from build123d import *

# Parameters (mm, degrees)
SKETCH1_R                        = 127
SKETCH1_R_2                      = 25.4
BOSS_EXTRUDE2_DEPTH              = 19.05
F_1_4_20_TAPPED_HOLE1_AT_2_COUNT = 2
F_1_4_20_TAPPED_HOLE1_AT_2_PITCH = 127
F_1_4_20_TAPPED_HOLE1_AT_3_COUNT = 2
F_1_4_20_TAPPED_HOLE1_AT_3_PITCH = 107.763073453
F_1_4_20_TAPPED_HOLE1_AT_4_COUNT = 2
F_1_4_20_TAPPED_HOLE1_AT_4_PITCH = 177.8
F_1_4_20_TAPPED_HOLE1_AT_5_COUNT = 2
F_1_4_20_TAPPED_HOLE1_AT_5_PITCH = 152.4
F_1_4_20_TAPPED_HOLE1_AT_6_COUNT = 2
F_1_4_20_TAPPED_HOLE1_AT_6_PITCH = 127
F_1_4_20_TAPPED_HOLE1_AT_7_COUNT = 2
F_1_4_20_TAPPED_HOLE1_AT_7_PITCH = 107.763073453
F_1_4_20_TAPPED_HOLE1_AT_8_COUNT = 2
F_1_4_20_TAPPED_HOLE1_AT_8_PITCH = 25.4


with BuildPart() as part:
    # Sketch1 → Boss-Extrude2 (new body)
    with BuildSketch(Plane.XY):
        Circle(SKETCH1_R)
        Circle(SKETCH1_R_2, mode=Mode.SUBTRACT)
    extrude(amount=BOSS_EXTRUDE2_DEPTH)

    # Sketch5 → 1/4-20 Tapped Hole1 (revolve, cut)
    with BuildSketch(Plane(origin=(-76.2, 0, 19.05), x_dir=(0, -1, 0), z_dir=(1, 0, 0))):
        Polygon((0, 0), (0, 19.05), (3.81, 19.05), (2.5527, 17.7927), (2.5527, 1.2573), (3.81, 0), align=None)
    f_1_4_20_tapped_hole1 = revolve(axis=Axis((-76.2, 0, 25.4), (0, 0, -1)), mode=Mode.SUBTRACT)

    # 1/4-20 Tapped Hole1 at 2: 1/4-20 Tapped Hole1 ×2
    with Locations(*[Vector(0.6, 0.8, 0) * (i * F_1_4_20_TAPPED_HOLE1_AT_2_PITCH) for i in range(1, F_1_4_20_TAPPED_HOLE1_AT_2_COUNT)]):
        add(f_1_4_20_tapped_hole1, mode=Mode.SUBTRACT)

    # 1/4-20 Tapped Hole1 at 3: 1/4-20 Tapped Hole1 ×2
    with Locations(*[Vector(0.707106781, 0.707106781, 0) * (i * F_1_4_20_TAPPED_HOLE1_AT_3_PITCH) for i in range(1, F_1_4_20_TAPPED_HOLE1_AT_3_COUNT)]):
        add(f_1_4_20_tapped_hole1, mode=Mode.SUBTRACT)

    # 1/4-20 Tapped Hole1 at 4: 1/4-20 Tapped Hole1 ×2
    with Locations(*[(i * F_1_4_20_TAPPED_HOLE1_AT_4_PITCH, 0, 0) for i in range(1, F_1_4_20_TAPPED_HOLE1_AT_4_COUNT)]):
        add(f_1_4_20_tapped_hole1, mode=Mode.SUBTRACT)

    # 1/4-20 Tapped Hole1 at 5: 1/4-20 Tapped Hole1 ×2
    with Locations(*[(i * F_1_4_20_TAPPED_HOLE1_AT_5_PITCH, 0, 0) for i in range(1, F_1_4_20_TAPPED_HOLE1_AT_5_COUNT)]):
        add(f_1_4_20_tapped_hole1, mode=Mode.SUBTRACT)

    # 1/4-20 Tapped Hole1 at 6: 1/4-20 Tapped Hole1 ×2
    with Locations(*[Vector(0.6, -0.8, 0) * (i * F_1_4_20_TAPPED_HOLE1_AT_6_PITCH) for i in range(1, F_1_4_20_TAPPED_HOLE1_AT_6_COUNT)]):
        add(f_1_4_20_tapped_hole1, mode=Mode.SUBTRACT)

    # 1/4-20 Tapped Hole1 at 7: 1/4-20 Tapped Hole1 ×2
    with Locations(*[Vector(0.707106781, -0.707106781, 0) * (i * F_1_4_20_TAPPED_HOLE1_AT_7_PITCH) for i in range(1, F_1_4_20_TAPPED_HOLE1_AT_7_COUNT)]):
        add(f_1_4_20_tapped_hole1, mode=Mode.SUBTRACT)

    # 1/4-20 Tapped Hole1 at 8: 1/4-20 Tapped Hole1 ×2
    with Locations(*[(-i * F_1_4_20_TAPPED_HOLE1_AT_8_PITCH, 0, 0) for i in range(1, F_1_4_20_TAPPED_HOLE1_AT_8_COUNT)]):
        add(f_1_4_20_tapped_hole1, mode=Mode.SUBTRACT)


solid = part.part
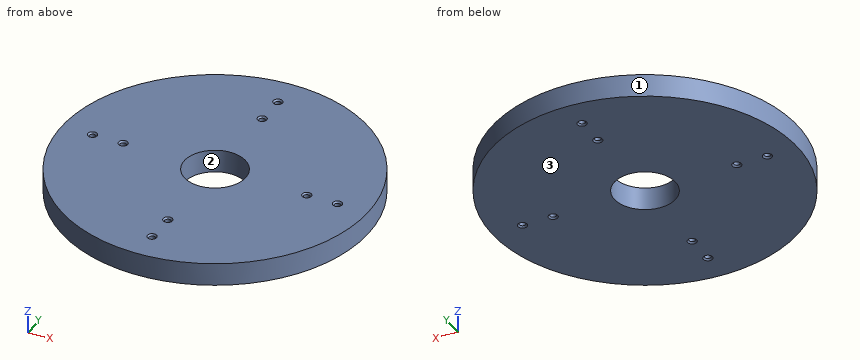
Check sheet for the modelled part. Datum: model origin and axes. Units: mm. Face numbers are marked on the shaded views. Round coordinates to 2 decimals unless told otherwise and drop trailing zeros. Loops run counter-clockwise (first coordinate to the right, second up) from the corner with the lowest first, then second, coordinate; pieces in that order, holes last. Notation, with made-up numbers: (35.5, 11) - (56.5, 11) arc R14 cw to (56.5, 26) - close; hole circle Ø6 at (-29, 26). An arc over 180 degrees is marked (long way). Answer as CSV lines item,"result". Start each with the question number.
Item 1: Release check for a two-part mould opening along Y. For the marked faces 1, 2 and 3 record: +Y half, -Y half, draft (parallel to the pull), parting line (faces both ways), or undercut.
Item 2: Scan lines: line 1 (Y direction, x = 0, z = 6.75); line 2 (X direction, y = 101.6, z = 6.25); line 3 (Y direction, x = 75, z = 13). Record each from-to range of solid material in increasing order. Write a range as [from, to].
Item 3: Section check C-C (y = 35). Record the boundary of the cut face in (x, z), and give its area (3 significant figures).
Item 4: Section check B-B (x = -22.5). Record the boundary of the cut face in (y, z).
Item 5: Section check A-A (z = 7.75). Count the separate pieces of the cut face and the enclosed holes in it, and give its area (3 significant figures).
Item 6: Depth check by flat-ended pin: P1, Ø6, axis at y = -40.5, z = 9.5, coming from the -X side; P2, Ø4, axis at x = -101.6, y = 0, coming from the +Z side; P3, Ø6.5, axis at x = 101.6, y = 0, coming from the -Z side; P4, Ø5, axis at x = 39.5, z = 3.5, coming from the -Y side. Enter the tip coordinate at first touch or a pass-through.
Report:
1,face 1,"parting line"
1,face 2,"undercut"
1,face 3,"draft"
2,line 1,"y = [-127, -104.15], [-99.05, -78.75], [-73.65, -25.4], [25.4, 73.65], [78.75, 99.05], [104.15, 127]"
2,line 2,"x = [-76.2, -2.55], [2.55, 76.2]"
2,line 3,"y = [-102.49, -2.25], [2.25, 102.49]"
3,outline,"(-122.08, 0) - (122.08, 0) - (122.08, 19.05) - (-122.08, 19.05) - close"
3,area,"4,650 mm2"
4,outline,"(-124.99, 0) - (-11.79, 0) - (-11.79, 19.05) - (-124.99, 19.05) - close; (11.79, 0) - (124.99, 0) - (124.99, 19.05) - (11.79, 19.05) - close"
5,separate pieces,"1"
5,enclosed holes,"9"
5,area,"48,500 mm2"
6,P1,"stops at x = -121.34"
6,P2,"passes through"
6,P3,"stops at z = 0.56"
6,P4,"stops at y = -121.49"
